Model file for the job. Use its own axes, mm. A direction names the side the tool comes from. Round coordinates to 2 decimals unless told otherwise and drop trailing zeros. Loops run counter-clockwise (first coordinate to the right, second up) from the corner with the lowest first, then second, coordinate; pieces in that order, holes last. Notation, with made-up numbers: M -38,18.25 L -6,18.25 A16 cw -6,39.25 Z; hole C 70.25,34.25 d8. An arc over 180 degrees is marked long. Answer in a Markdown table with one row per item.
from build123d import *

# Parameters (mm, degrees)
SKETCH_1_R      = 65
EXTRUDE_1_DEPTH = 50
SKETCH_2_R      = 65
SKETCH_2_R_2    = 60
EXTRUDE_2_DEPTH = 60
SKETCH_3_R      = 100
EXTRUDE_3_DEPTH = 10
FILLET_1_R      = 30


with BuildPart() as part:
    # 草图1 → 凸台-拉伸1 (new body)
    with BuildSketch(Plane(origin=(0, 0, 0), x_dir=(1, 0, 0), z_dir=(0, 1, 0))):
        with Locations(Location((0, 0, 0), (0, 0, 270))):
            Circle(SKETCH_1_R)
    extrude(amount=EXTRUDE_1_DEPTH)

    # 草图2 → 凸台-拉伸2 (add)
    with BuildSketch(Plane(origin=(0, 50, 0), x_dir=(1, 0, 0), z_dir=(0, 1, 0))):
        with Locations(Location((0, 0, 0), (0, 0, 270))):
            Circle(SKETCH_2_R)
        with Locations(Location((0, 0, 0), (0, 0, 270))):
            Circle(SKETCH_2_R_2, mode=Mode.SUBTRACT)
    extrude(amount=EXTRUDE_2_DEPTH)

    # 草图3 → 凸台-拉伸3 (add)
    with BuildSketch(Plane.XZ):
        with Locations(Location((0, 0, 0), (0, 0, 270))):
            Circle(SKETCH_3_R)
    extrude(amount=EXTRUDE_3_DEPTH)

    # 圆角1
    fillet_1_edges = [part.edges().sort_by_distance(p)[0] for p in [
        (0, 0, -65),
    ]]
    fillet(fillet_1_edges, radius=FILLET_1_R)


solid = part.part
1. Wall check: probe 1 along X at (y, z) = (78, 0); probe 2 along Z at (x, y) = (31.5, 71); probe 3 along X at (y, z) = (73, -29.5). Give the ranges that are in metal, low to high.
Verdict:
| item | result |
|---|---|
| probe 1 | x = -65 to -60, 60 to 65 |
| probe 2 | z = -56.86 to -51.07, 51.07 to 56.86 |
| probe 3 | x = -57.92 to -52.25, 52.25 to 57.92 |
2. Saw through at C-C (y = 67). Write the cut outline in (x, z), and give its area (3 significant figures).
Verdict:
| item | result |
|---|---|
| outline | C 0,0 d130; hole C 0,0 d120 |
| area | 1,960 mm² |
3. Saw through at B-B (z = 0). Write the cut outline in (x, y), and give its area (3 significant figures).
Verdict:
| item | result |
|---|---|
| outline | M -100,-10 L 100,-10 L 100,0 L 95,0 A30 cw 65,30 L 65,110 L 60,110 L 60,50 L -60,50 L -60,110 L -65,110 L -65,30 A30 cw -95,0 L -100,0 Z |
| area | 9,490 mm² |
4. Mould opens along X. For faces 3 (the cylindrical face through (2.64, 79.58, -59.94)), 4 (the cylindrical face through (30.04, -4.93, -95.38)), 5 (the flat face through (-37, 0, -88)) say: +X half, -X half, draft (parallel to the pull), parting line (faces both ways), or undercut.
Verdict:
| item | result |
|---|---|
| face 3 | undercut |
| face 4 | parting line |
| face 5 | draft |
5. Pin check, flat tips, straight feed: pin 1 (8 mm diameter, centred on x = 31.5, y = 51.5, fed in from -Z); pin 2 (1.5 mm diameter, centred on x = 53, y = 39.5, fed in from +Z); pin 3 (12 mm diameter, centred on y = 59.5, z = 62, fed in from -X). Stop position of each tip, or through.
Verdict:
| item | result |
|---|---|
| pin 1 | stops at z = -58.9 |
| pin 2 | stops at z = 38.66 |
| pin 3 | stops at x = -33 |
6. Tool access for faces 1 (the flat face through (1, 50, -1)), 2 (the flat face through (-57.5, 110, 19)): list every direction of +Z, -Z, +X, -X, +Y, -Y with a clear straight run to the whole face (end or side of a thin tool).
Verdict:
| item | result |
|---|---|
| face 1 | +Y |
| face 2 | +Z, -Z, +X, -X, +Y |
7. Saw through at A-A (x = 0). Write the cut outline in (y, z), and give its area (3 significant figures).
Verdict:
| item | result |
|---|---|
| outline | M -10,-100 L 0,-100 L 0,-95 A30 cw 30,-65 L 110,-65 L 110,-60 L 50,-60 L 50,60 L 110,60 L 110,65 L 30,65 A30 cw 0,95 L 0,100 L -10,100 Z |
| area | 9,490 mm² |
